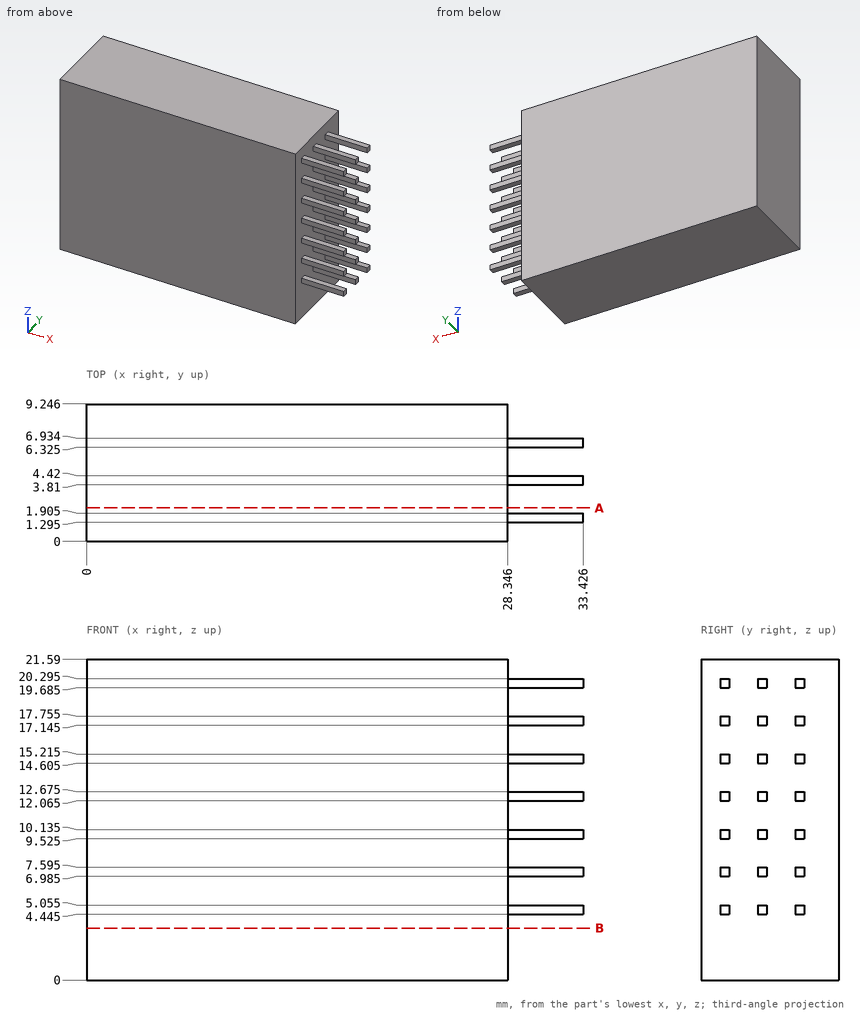
Design review of the part shown in the three views and the two pictorial views. Dimensions are in mm from the part's minimum x, y and z. Round coordinates to 2 decimals unless told otherwise and drop trailing zeros. Loops run counter-clockwise (first coordinate to the right, second up) from the corner with the lowest first, then second, coordinate; pieces in that order, holes last. Notation, with made-up numbers: M 47,23.25 L 80,23.25 A15 ccw 80,38.25 Z; hole C 80.5,41.5 d9. An arc over 180 degrees is marked long. Write item = value, one per line.
Item 1: Insertion check: P1, Ø0.5, axis at x = 30.5, z = 17.5, coming from the +Y side; P2, Ø1, axis at y = 4.5, z = 18.5, coming from the -X side; P3, Ø0.5, axis at x = 31, y = 6.5, coming from the -Z side (3 decimals); P4, Ø0.7, axis at x = 30.5, z = 4.5, coming from the -Y side (1 decimal). Each pin has a flat end and moves straight along its axis. Give the tip position at first contact, or say it passes through.
Return value:
P1 = 6.93
P2 = 0
P3 = 4.445
P4 = 1.3
Item 2: Take a section at A-A on y = 2.25. Write out the cut boundary in (x, z).
Return value:
outline = M 0,0 L 28.35,0 L 28.35,21.59 L 0,21.59 Z
Item 3: Take a section at B-B on z = 3.5. Write out the cut boundary in (x, y) (1 decimal), then the cut area to 3 significant figures.
Return value:
outline = M 0,0 L 28.3,0 L 28.3,9.2 L 0,9.2 Z
area = 262 mm2
Item 4: For line 1 (X direction, y = 1, z = 5.25), list the stretches that pass through material, from the lowest coordinate up. Write a range as [from, to].
Return value:
line_1 = [0, 28.35]
